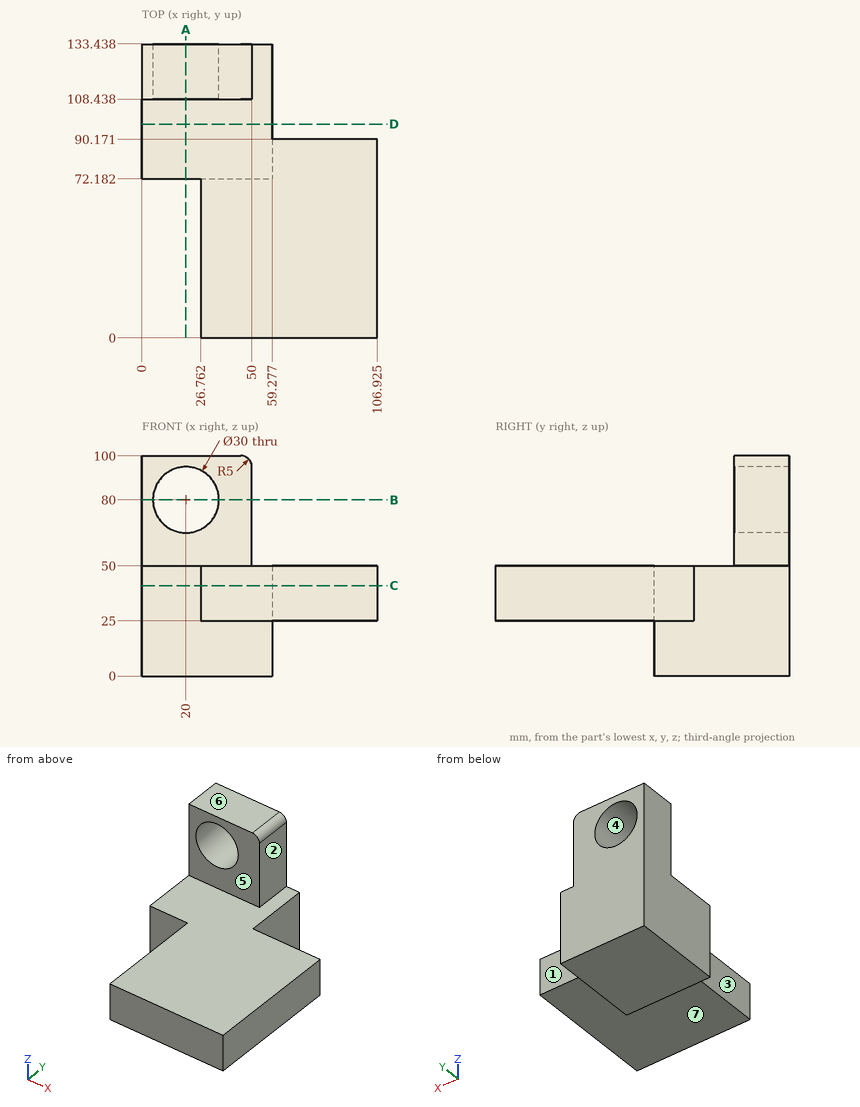
Here's the drawing with two shaded views (mm, measured from the low corner). I have some questions. A direction names the side the tool comes from. Give positions to 0.01 mm unless a question says otherwise; leave off trailing zeros. Order: outer loops, then holes, each group sorted by start corner. A loop starts at its lowest first (then second) coordinate and runs counter-clockwise, first axis right, second up.
Q1. Suppose I cut it at D-D, the plane y = 97. Write out the boundary of the cut face in (x, z).
Q2. Suppose I cut it at C-C, the plane z = 41. Write out the boundary of the cut face in (x, y) (1 decimal), and give its area (3 significant figures).
Q3. For the marked faces 5, 6 and 7, which set-ups out of +Z, -Z, +X, -X, +Y, -Y let a thin tool reach every point of the face, with its end or its side?
Q4. Suppose I cut it at B-B, the plane z = 80. Write out the boundary of the cut face in (x, y), and give its area (3 significant figures).
Q5. I'm going to push flat-ended pins straight in: P1, Ø20, axis at y = 38.5, z = 40, coming from the -X side; P2, Ø3, axis at x = 80.5, y = 54.5, coming from the +Z side; P3, Ø24, axis at x = 75.5, y = 61, coming from the -Z side. Where does each tip first touch, or does it pass through?
Q6. We'd pull the mould along X, two halves only. Please class the marked faces 1, 2, 3 and 4: +X half, -X half, draft (parallel to the pull), parting line (faces both ways), or undercut.
Q7. If I drill on line 1 along Z through (x, y) = (20, 116.5); line 2 along Y through (x, z) = (64, 45); line 3 along X through (y, z) = (42.5, 35) (1 decimal), over which ranges is the centre line in solid material (lowest first)?
Q8. Suppose I cut it at A-A, the plane x = 20. Write out the boundary of the cut face in (y, z), and give its area (3 significant figures).
Solution:
1. outline: (0, 0) - (59.28, 0) - (59.28, 50) - (0, 50) - close
2. outline: (0, 72.2) - (26.8, 72.2) - (26.8, 0) - (106.9, 0) - (106.9, 90.2) - (59.3, 90.2) - (59.3, 133.4) - (0, 133.4) - close
2. area: 10,300 mm2
3. face 5: +Z, +X, -X, -Y
3. face 6: +Z, +X, -X, +Y, -Y
3. face 7: -Z, +X, -Y
4. outline: (0, 108.44) - (5, 108.44) - (5, 133.44) - (0, 133.44) - close; (35, 108.44) - (50, 108.44) - (50, 133.44) - (35, 133.44) - close
4. area: 500 mm2
5. P1: stops at x = 26.76
5. P2: stops at z = 50
5. P3: stops at z = 25
6. face 1: draft
6. face 2: +X half
6. face 3: -X half
6. face 4: undercut
7. line 1: z = 0 to 65, 95 to 100
7. line 2: y = 0 to 90.17
7. line 3: x = 26.8 to 106.9
8. outline: (72.18, 0) - (133.44, 0) - (133.44, 65) - (108.44, 65) - (108.44, 50) - (72.18, 50) - close; (108.44, 95) - (133.44, 95) - (133.44, 100) - (108.44, 100) - close
8. area: 3,560 mm2
